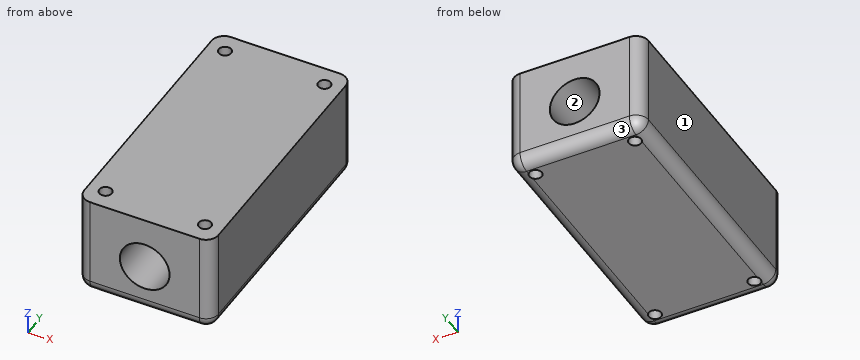
from build123d import *

# Parameters (mm, degrees)
F0_W         = 54
F0_H         = 41
F0_R         = 10
F1_DEPTH     = 106
F3_D         = 5
F4_T1_DEPTH  = 48.5
F4_T3_DEPTH  = 44
F4_T5_DEPTH  = 96
F4_S9_W      = 5
F4_S9_H      = 5
F4_T10_DEPTH = 5
F4_S15_W     = 5
F4_S15_H     = 5
F4_T16_DEPTH = 5
F4_S21_W     = 5
F4_S21_H     = 5
F4_T22_DEPTH = 5
F4_S27_W     = 5
F4_S27_H     = 5
F4_T28_DEPTH = 5


# Not quite as in the source:
# - a fillet or chamfer that OpenCascade refuses, or shapes differently, is made with other operations: its cross-section is extruded or revolved along the edge and cut away or added


with BuildPart() as f1:
    # F0 (on Front) → F1 (new body)
    with BuildSketch(Plane.XZ):
        Rectangle(F0_W, F0_H)
        with Locations((0, -0.5)):
            Circle(F0_R, mode=Mode.SUBTRACT)
    extrude(amount=F1_DEPTH)

    # F3 (through all)
    with Locations(Plane.XY.offset(20.5)):
        with Locations((-20, -8), (20, -8), (-20, -98), (20, -98)):
            Hole(F3_D / 2)

    # F4: fillet of radius 5 on 8 edges, made by hand

    # F4_s2 → F4_t1 (cut)
    with BuildSketch(Plane.XY.offset(-15.5)):
        with BuildLine():
            ThreePointArc((-22, -106), (-25.5355339059, -104.5355339059), (-27, -101))
            Line((-27, -101), (-27, -106))
            Line((-27, -106), (-22, -106))
        make_face()
        with BuildLine():
            ThreePointArc((27, -101), (25.5355339059, -104.5355339059), (22, -106))
            Line((22, -106), (27, -106))
            Line((27, -106), (27, -101))
        make_face()
        with BuildLine():
            ThreePointArc((27, -5), (25.5355339059, -1.4644660941), (22, 0))
            Line((22, 0), (27, 0))
            Line((27, 0), (27, -5))
        make_face()
        with BuildLine():
            ThreePointArc((-22, 0), (-25.5355339059, -1.4644660941), (-27, -5))
            Line((-27, -5), (-27, 0))
            Line((-27, 0), (-22, 0))
        make_face()
    extrude(amount=F4_T1_DEPTH, mode=Mode.SUBTRACT)

    # F4_s4 → F4_t3 (cut)
    with BuildSketch(Plane.YZ.offset(-22)):
        with BuildLine():
            ThreePointArc((-101, -20.5), (-104.5355339059, -19.0355339059), (-106, -15.5))
            Line((-106, -15.5), (-106, -20.5))
            Line((-106, -20.5), (-101, -20.5))
        make_face()
        with BuildLine():
            ThreePointArc((-5, -20.5), (-1.4644660941, -19.0355339059), (0, -15.5))
            Line((0, -15.5), (0, -20.5))
            Line((0, -20.5), (-5, -20.5))
        make_face()
    extrude(amount=F4_T3_DEPTH, mode=Mode.SUBTRACT)

    # F4_s6 → F4_t5 (cut)
    with BuildSketch(Plane.XZ.offset(5)):
        with BuildLine():
            ThreePointArc((27, -15.5), (25.5355339059, -19.0355339059), (22, -20.5))
            Line((22, -20.5), (27, -20.5))
            Line((27, -20.5), (27, -15.5))
        make_face()
        with BuildLine():
            ThreePointArc((-22, -20.5), (-25.5355339059, -19.0355339059), (-27, -15.5))
            Line((-27, -15.5), (-27, -20.5))
            Line((-27, -20.5), (-22, -20.5))
        make_face()
    extrude(amount=F4_T5_DEPTH, mode=Mode.SUBTRACT)


with BuildPart() as f4_tool8:
    # F4_s9 → F4_t10 (new body)
    with BuildSketch(Plane.XY.offset(-15.5)):
        with Locations((-24.5, -103.5)):
            Rectangle(F4_S9_W, F4_S9_H)
    extrude(amount=-F4_T10_DEPTH)

    # F4_s11 → F4_t12 (revolve, cut)
    with BuildSketch(Plane(origin=(-22, -101, -15.5), x_dir=(0.7071067812, 0.7071067812, 0), z_dir=(-0.7071067812, 0.7071067812, 0))):
        with BuildLine():
            ThreePointArc((0, -5), (5, 0), (0, 5))
            Line((0, 5), (0, -5))
        make_face()
    revolve(axis=Axis((-22, -101, -15.5), (0, 0, -1)), mode=Mode.SUBTRACT)


with BuildPart() as f1_1:
    add(f1.part)

    # F4_t7: cut F4_tool8
    add(f4_tool8.part, mode=Mode.SUBTRACT)


with BuildPart() as f4_tool14:
    # F4_s15 → F4_t16 (new body)
    with BuildSketch(Plane.YZ.offset(22)):
        with Locations((-103.5, -18)):
            Rectangle(F4_S15_W, F4_S15_H)
    extrude(amount=F4_T16_DEPTH)

    # F4_s17 → F4_t18 (revolve, cut)
    with BuildSketch(Plane(origin=(22, -101, -15.5), x_dir=(0, 0.7071067812, 0.7071067812), z_dir=(0, 0.7071067812, -0.7071067812))):
        with BuildLine():
            ThreePointArc((0, -5), (5, 0), (0, 5))
            Line((0, 5), (0, -5))
        make_face()
    revolve(axis=Axis((22, -101, -15.5), (1, 0, 0)), mode=Mode.SUBTRACT)


with BuildPart() as f1_2:
    add(f1_1.part)

    # F4_t13: cut F4_tool14
    add(f4_tool14.part, mode=Mode.SUBTRACT)


with BuildPart() as f4_tool20:
    # F4_s21 → F4_t22 (new body)
    with BuildSketch(Plane.YZ.offset(22)):
        with Locations((-2.5, -18)):
            Rectangle(F4_S21_W, F4_S21_H)
    extrude(amount=F4_T22_DEPTH)

    # F4_s23 → F4_t24 (revolve, cut)
    with BuildSketch(Plane(origin=(22, -5, -15.5), x_dir=(0, -0.7071067812, 0.7071067812), z_dir=(0, 0.7071067812, 0.7071067812))):
        with BuildLine():
            ThreePointArc((0, -5), (5, 0), (0, 5))
            Line((0, 5), (0, -5))
        make_face()
    revolve(axis=Axis((22, -5, -15.5), (1, 0, 0)), mode=Mode.SUBTRACT)


with BuildPart() as f1_3:
    add(f1_2.part)

    # F4_t19: cut F4_tool20
    add(f4_tool20.part, mode=Mode.SUBTRACT)


with BuildPart() as f4_tool26:
    # F4_s27 → F4_t28 (new body)
    with BuildSketch(Plane.XY.offset(-15.5)):
        with Locations((-24.5, -2.5)):
            Rectangle(F4_S27_W, F4_S27_H)
    extrude(amount=-F4_T28_DEPTH)

    # F4_s29 → F4_t30 (revolve, cut)
    with BuildSketch(Plane(origin=(-22, -5, -15.5), x_dir=(0.7071067812, -0.7071067812, 0), z_dir=(0.7071067812, 0.7071067812, 0))):
        with BuildLine():
            ThreePointArc((0, -5), (5, 0), (0, 5))
            Line((0, 5), (0, -5))
        make_face()
    revolve(axis=Axis((-22, -5, -15.5), (0, 0, -1)), mode=Mode.SUBTRACT)


with BuildPart() as f1_4:
    add(f1_3.part)

    # F4_t25: cut F4_tool26
    add(f4_tool26.part, mode=Mode.SUBTRACT)


solid = f1_4.part
Source: CAD feature listing. Evaluate the final solid. Frame: model axes, mm. Face numbers are marked on the shaded views. Coordinates: 2 decimals unless noted, no trailing zeros. Loops run counter-clockwise (first coordinate to the right, second up) from the corner with the lowest first, then second, coordinate; pieces in that order, holes last. Notation, with made-up numbers: (54, 34.5) - (85, 34.5) arc R28 ccw to (85, 73.5) - close; hole circle Ø6 at (15, -22.5). An arc over 180 degrees is marked (long way). One line per item, written item: value. Start each with the question number.
1. Mould query, pull axis X, two halves, no side actions, for the marked faces 1, 2 and 3. Classes: pulls with the +X half, pulls with the -X half, needs draft (parallel to the pull), parting line crosses it, or undercut.
2. Contact query for a flat-ended pin moving along its axis: P1, Ø4, axis at x = -20, y = -8, coming from the +Z side. Output: stop coordinate, or through.
3. Section D-D (x = 0). Return the cut outline in (y, z), and give its area (3 significant figures).
4. Section C-C (z = 15). Return the cut outline in (x, y).
5. Ray query, L1, parallel to Y at x = 20, z = -10; L2, parallel to Y at x = 21, z = -6; L3, parallel to X at y = -98, z = 5. Return the intervals inside material, ascending.
6. Section A-A (z = -0.5). Return the cut outline in (x, y).
7. Section B-B (x = 20). Return the cut outline in (y, z).
Verdict:
1. face 1: pulls with the -X half
1. face 2: undercut
1. face 3: needs draft
2. P1: passes through
3. outline: (-106, -15.5) arc R5 ccw to (-101, -20.5) - (-5, -20.5) arc R5 ccw to (0, -15.5) - (0, -10.5) - (-106, -10.5) - close; (-106, 9.5) - (0, 9.5) - (0, 20.5) - (-106, 20.5) - close
3. area: 2,220 mm2
4. outline: (-27, -101) arc R5 ccw to (-22, -106) - (22, -106) arc R5 ccw to (27, -101) - (27, -5) arc R5 ccw to (22, 0) - (-22, 0) arc R5 ccw to (-27, -5) - close; hole circle Ø5 at (-20, -98); hole circle Ø5 at (-20, -8); hole circle Ø5 at (20, -98); hole circle Ø5 at (20, -8)
5. L1: y = -106 to -100.5, -95.5 to -10.5, -5.5 to 0
5. L2: y = -106 to -100.29, -95.71 to -10.29, -5.71 to 0
5. L3: x = -27 to -22.5, -17.5 to -8.35, 8.35 to 17.5, 22.5 to 27
6. outline: (-27, -101) arc R5 ccw to (-22, -106) - (-10, -106) - (-10, 0) - (-22, 0) arc R5 ccw to (-27, -5) - close; (10, -106) - (22, -106) arc R5 ccw to (27, -101) - (27, -5) arc R5 ccw to (22, 0) - (10, 0) - close; hole circle Ø5 at (-20, -98); hole circle Ø5 at (-20, -8); hole circle Ø5 at (20, -98); hole circle Ø5 at (20, -8)
7. outline: (-106, -15.5) arc R5 ccw to (-101, -20.5) - (-100.5, -20.5) - (-100.5, 20.5) - (-106, 20.5) - close; (-95.5, -20.5) - (-10.5, -20.5) - (-10.5, 20.5) - (-95.5, 20.5) - close; (-5.5, -20.5) - (-5, -20.5) arc R5 ccw to (0, -15.5) - (0, 20.5) - (-5.5, 20.5) - close
